Autodesk Inventor part; units mm, degrees
ref_plane "YZ Plane" through (0, 0, 0) normal (1, 0, 0) x (0, 1, 0)
ref_plane "XZ Plane" through (0, 0, 0) normal (0, 1, 0) x (-1, 0, 0)
ref_plane "XY Plane" through (0, 0, 0) normal (0, 0, 1) x (1, 0, 0)
sketch "Sketch1" plane through (0, 0, 0) normal (0, 0, 1) x (1, 0, 0)
  line L0 (-32.5, 32.5) -> (32.5, 32.5) construction
  line L1 (32.5, 32.5) -> (32.5, -32.5) construction
  line L2 (32.5, -32.5) -> (-32.5, -32.5) construction
  line L3 (-32.5, -32.5) -> (-32.5, 32.5) construction
  circle A0 centre (-32.5, 32.5) radius 2.5
  circle A1 centre (32.5, 32.5) radius 2.5
  circle A2 centre (-32.5, -32.5) radius 2.5
  circle A3 centre (32.5, -32.5) radius 2.5
  line L4 (-32.5, 32.5) -> (32.5, -32.5) construction
  circle A4 centre (0, 0) radius 12.5
  circle A5 centre (-32.5, 32.5) radius 4.25
  circle A6 centre (32.5, 32.5) radius 4.25
  circle A7 centre (-32.5, -32.5) radius 4.25
  circle A8 centre (32.5, -32.5) radius 4.25
  line L5 (-32.5, 36.75) -> (32.5, 36.75)
  line L6 (32.5, -36.75) -> (-32.5, -36.75)
  line L7 (-36.75, 32.5) -> (-36.75, -32.5)
  line L8 (36.75, 32.5) -> (36.75, -32.5)
  dimension "d1" = 65
  dimension "d2" = 5
  dimension "d4" = 25
  dimension "d16" = 8.5
extrude "Extrusion1" add sketch "Sketch1" along normal blind 3
sketch "Sketch2" plane through (0, 0, 3) normal (0, 0, 1) x (1, 0, 0)
  line L0 (-17.55, 17.55) -> (17.55, 17.55)
  line L1 (17.55, -17.55) -> (-17.55, -17.55)
  line L2 (0, 17.55) -> (0, 36.75) construction
  line L3 (0, -17.55) -> (0, -36.75) construction
  line L4 (-19.55, 19.55) -> (19.55, 19.55)
  line L5 (19.55, -19.55) -> (-19.55, -19.55)
  line L6 (17.55, 17.55) -> (19.55, 19.55) construction
  line L7 (-17.55, 17.55) -> (-19.55, 19.55) construction
  line L8 (-19.55, -19.55) -> (-17.55, -17.55) construction
  line L9 (17.55, -17.55) -> (19.55, -19.55) construction
  circle A0 centre (0, 0) radius 12.5
  circle A1 centre (-32.5, -32.5) radius 2.5
  circle A2 centre (32.5, -32.5) radius 2.5
  circle A3 centre (32.5, 32.5) radius 2.5
  circle A4 centre (-32.5, 32.5) radius 2.5
  arc A5 (32.5, -36.75) -> (36.75, -32.5) centre (32.5, -32.5) ccw
  line L10 (36.75, -32.5) -> (36.75, 32.5)
  arc A6 (36.75, 32.5) -> (32.5, 36.75) centre (32.5, 32.5) ccw
  line L11 (32.5, 36.75) -> (-32.5, 36.75)
  arc A7 (-32.5, 36.75) -> (-36.75, 32.5) centre (-32.5, 32.5) ccw
  line L12 (-36.75, 32.5) -> (-36.75, -32.5)
  arc A8 (-36.75, -32.5) -> (-32.5, -36.75) centre (-32.5, -32.5) ccw
  line L13 (-32.5, -36.75) -> (32.5, -36.75)
  line L14 (-32.5, -36.75) -> (32.5, -36.75)
  line L15 (36.75, -32.5) -> (36.75, 32.5)
  line L16 (32.5, 36.75) -> (-32.5, 36.75)
  line L17 (-19.55, 12.5) -> (-17.55, 12.5)
  line L18 (-19.55, -12.5) -> (-17.55, -12.5)
  line L19 (-19.55, -19.55) -> (-19.55, -12.5)
  line L20 (-19.55, 12.5) -> (-19.55, 19.55)
  line L21 (-17.55, -17.55) -> (-17.55, -12.5)
  line L22 (-17.55, 12.5) -> (-17.55, 17.55)
  line L23 (17.55, 12.5) -> (19.55, 12.5)
  line L24 (17.55, -12.5) -> (19.55, -12.5)
  line L25 (17.55, 17.55) -> (17.55, 12.5)
  line L26 (17.55, -12.5) -> (17.55, -17.55)
  line L27 (19.55, 19.55) -> (19.55, 12.5)
  line L28 (19.55, -12.5) -> (19.55, -19.55)
  line L29 (-17.55, 17.55) -> (0, 0) construction
  line L30 (0, 0) -> (-17.55, -17.55) construction
  line L31 (0, 0) -> (17.55, 17.55) construction
  line L32 (0, 0) -> (17.55, -17.55) construction
  dimension "d7" = 35.1
  dimension "d23" = 25
  dimension "d24" = 2
  dimension "d31" = 2
extrude "Extrusion2" add sketch "Sketch2" along normal blind 2 contours L22 L17 L20 L4 L27 L23 L25 L0 | L26 L24 L28 L5 L19 L18 L21 L1
extrude "Extrusion4" add sketch "Sketch1" along normal blind 6 contours A5 | A6 | A7 | A8
sketch "Sketch4" plane through (0, 0, 3) normal (0, 0, 1) x (1, 0, 0)
  line L0 (19.55, 19.55) -> (19.55, 12.5)
  line L1 (-19.55, 19.55) -> (19.55, 19.55)
  arc A0 (36.75, -32.5) -> (32.5, -36.75) centre (32.5, -32.5) ccw
  line L2 (36.75, -32.5) -> (36.75, 32.5)
  arc A1 (32.5, 36.75) -> (36.75, 32.5) centre (32.5, 32.5) ccw
  line L3 (32.5, 36.75) -> (-32.5, 36.75)
  arc A2 (-36.75, 32.5) -> (-32.5, 36.75) centre (-32.5, 32.5) ccw
  line L4 (-36.75, 32.5) -> (-36.75, -32.5)
  arc A3 (-32.5, -36.75) -> (-36.75, -32.5) centre (-32.5, -32.5) ccw
  line L5 (-32.5, -36.75) -> (32.5, -36.75)
  line L6 (-19.55, 14) -> (-19.55, -14)
  line L7 (-19.55, -14) -> (-36.75, -14)
  line L8 (-36.75, -14) -> (-36.75, 14)
  line L9 (-36.75, 14) -> (-19.55, 14)
  line L10 (32.5, 36.75) -> (-32.5, 36.75) construction
  line L11 (0, 36.75) -> (0, -36.75) construction
  line L12 (19.55, 14) -> (19.55, -14)
  line L13 (19.55, -14) -> (36.75, -14)
  line L14 (36.75, -14) -> (36.75, 14)
  line L15 (36.75, 14) -> (19.55, 14)
  line L16 (-17.55, 17.55) -> (-17.55, 12.5)
  line L17 (-17.55, 12.5) -> (-19.55, 12.5)
  line L18 (-19.55, 12.5) -> (-19.55, 19.55)
  line L19 (19.55, 12.5) -> (17.55, 12.5)
  line L20 (17.55, 12.5) -> (17.55, 17.55)
  line L21 (17.55, 17.55) -> (-17.55, 17.55)
  point P0 (0, 0)
  point P1 (-36.75, 0)
  point P2 (36.75, 0)
  dimension "d20" = 28
extrude "Extrusion5" cut sketch "Sketch4" against normal through all contours L15 L2 L13 L12 L0 | L6 L7 L4 L9
sketch "Sketch5" plane through (0, 0, 5) normal (0, 0, 1) x (1, 0, 0)
  point P0 (0, 0)
properties part number "35mm glass cuvette holder"
CAD build for the part. Positions are in the model's coordinates, mm. A direction names the side the tool comes from. Round coordinates to 2 decimals unless told otherwise and drop trailing zeros. Write each loop counter-clockwise with the first axis right and the second up, starting at its lowest first coordinate (ties: lowest second). Pieces come first, ordered by that corner, then holes. Notation, with made-up numbers: (52.25, 43.5) - (111.25, 43.5) arc R27 ccw to (111.25, 74.5) - close; hole circle Ø11 at (-28.5, 66). An arc over 180 degrees is marked (long way). Write item = value, one per line. Start each with the question number.
Q1. Probe L1, parallel to Y at x = -32.5, z = 3.5; L2, parallel to Y at x = -32.5, z = 2.7; L3, parallel to Y at x = 0, z = 1.45. List the from-to ranges inside material, lowest first. Write a range as from..to.
Q2. Band-saw the part on C-C (y = 2). Give the cut face in (x, z).
Q3. Drop flat-ended pins along their axis: pin 1 (2 mm diameter, centred on x = 6, z = 4.5, fed in from +Y); pin 2 (7 mm diameter, centred on x = -8.5, y = 30.5, fed in from +Z); pin 3 (6 mm diameter, centred on x = -6.5, y = 4, fed in from -Z); pin 4 (18 mm diameter, centred on x = 7.5, y = -28.5, fed in from +Z). Give the stop position or say it passes through.
Q4. Mould opens along Y. For faces 1 (the flat face through (0, 17.55, 4)), 2 (the flat face through (35.3, -32.4, 6)), 3 (the flat face through (19.55, 0, 2)), 4 (the flat face through (0, -19.55, 4)) say: pulls with the +Y half, pulls with the -Y half, needs draft (parallel to the pull), parting line crosses it, or undercut.
Q5. Band-saw the part on B-B (z = 1). Give the cut face in (x, y).
Q6. Band-saw the part on A-A (x = 0). Give the cut face in (y, z).
Q7. Which spindle directions (+Z, -Z, +X, -X, +Y, -Y) get a long thin tool onto all of the face, cutting with end or side? Do faces 5 (the cylindrical face through (-34.34, -34.19, 2.96)), 6 (the flat face through (-19, -12.5, 4)), 7 (the cylindrical face through (-35.632, -35.372, 3.625)), 8 (the flat face through (28, 14, 2)), 9 (the flat face through (-29.7, 32.6, 6)). Say none if no direction does.
Q8. Band-saw the part on D-D (y = 16). Give the cut face in (x, z).
Answers below:
q1.L1 = -36.75..-35, -30..-28.25, 28.25..30, 35..36.75
q1.L2 = -36.75..-35, -30..-14, 14..30, 35..36.75
q1.L3 = -36.75..-12.5, 12.5..36.75
q2.outline = (-19.55, 0) - (-12.34, 0) - (-12.34, 3) - (-19.55, 3) - close; (12.34, 0) - (19.55, 0) - (19.55, 3) - (12.34, 3) - close
q3.pin_1 = 19.55
q3.pin_2 = 3
q3.pin_3 = through
q3.pin_4 = 5
q4.face_1 = undercut
q4.face_2 = needs draft
q4.face_3 = undercut
q4.face_4 = pulls with the -Y half
q5.outline = (-36.75, -32.5) arc R4.25 ccw to (-32.5, -36.75) - (32.5, -36.75) arc R4.25 ccw to (36.75, -32.5) - (36.75, -14) - (19.55, -14) - (19.55, 14) - (36.75, 14) - (36.75, 32.5) arc R4.25 ccw to (32.5, 36.75) - (-32.5, 36.75) arc R4.25 ccw to (-36.75, 32.5) - (-36.75, 14) - (-19.55, 14) - (-19.55, -14) - (-36.75, -14) - close; hole circle Ø5 at (-32.5, -32.5); hole circle Ø5 at (-32.5, 32.5); hole circle Ø25 at (0, 0); hole circle Ø5 at (32.5, -32.5); hole circle Ø5 at (32.5, 32.5)
q6.outline = (-36.75, 0) - (-12.5, 0) - (-12.5, 3) - (-17.55, 3) - (-17.55, 5) - (-19.55, 5) - (-19.55, 3) - (-36.75, 3) - close; (12.5, 0) - (36.75, 0) - (36.75, 3) - (19.55, 3) - (19.55, 5) - (17.55, 5) - (17.55, 3) - (12.5, 3) - close
q7.face_5 = +Z, -Z
q7.face_6 = +Z, +X, -X
q7.face_7 = +Z
q7.face_8 = +Z, -Z, +X
q7.face_9 = +Z, +X, -X, +Y, -Y
q8.outline = (-36.75, 0) - (36.75, 0) - (36.75, 3) - (19.55, 3) - (19.55, 5) - (17.55, 5) - (17.55, 3) - (-17.55, 3) - (-17.55, 5) - (-19.55, 5) - (-19.55, 3) - (-36.75, 3) - close
